Design review of the part built by this model. Coordinates are the model's own, in mm. A direction names the side the tool comes from. Round coordinates to 2 decimals unless told otherwise and drop trailing zeros. Order: outer loops, then holes, each group sorted by start corner. A loop starts at its lowest first (then second) coordinate and runs counter-clockwise, first axis right, second up. Notation, with made-up numbers: M 41,45.5 L 80,45.5 A26 ccw 80,65.5 Z; hole C 85.5,-5 d7. An arc over 180 degrees is marked long. Use a Markdown table: item, result. Add a question column.
(1) Take a section at A-A (z = -232.5). Write out the cut boundary in (x, y), then the cut area to 3 significant figures.
(2) Machinability: for faces 4 (the face through (0.986, 5.768, -155.615)), 5 (the face through (2, -11, -148)), which of the approach directions +Z, -Z, +X, -X, +Y, -Y give a long, thin tool a straight path to every point of the face, cutting with its end or side? Answer none if there is none.
(3) The part is to be moulded in two halves that separate along Z. For faces 1 (the face through (0.99, 24, -317.23)), 2 (the face through (0, -11, -148)), 3 (the face through (0.99, 27.33, -155.99)), say which applies: released by +Z, released by -Z, zero draft, split by the parting line, or undercut.
(4) To check wall thickness, follow probe 1 along Y at (x, z) = (1.9, -175.5); probe 2 along Z at (x, y) = (1.1, 35); probe 3 along Z at (x, y) = (1.9, -18.5). State the ranges of each line that lie inside material, in increasing order. Write a range as from..to.
(5) For pin 1 (0.6 mm diameter, centred on x = 1, y = -8, fed in from +Z); pin 2 (0.6 mm diameter, centred on x = 1, y = -49.5, fed in from -Z); pin 3 (0.6 mm diameter, centred on x = 1, z = -118.5, fed in from -Y), all flat-tipped, find the tip position at first contact; note any pin that passes through.
(6) Take a section at B-B (z = -116). Write out the cut boundary in (x, y), then the cut area to 3 significant figures.
(7) Take a section at C-C (x = 1.7). Count the separate pieces of the cut face and the enclosed holes in it, then the cut area to 3 significant figures.
```python
from build123d import *

# Parameters (mm, degrees)
SKETCH_1_W          = 40
SKETCH_1_H          = 2
SKETCH_1_W_2        = 50
SKETCH_1_R          = 15
SKETCH_1_W_3        = 30
SKETCH_1_W_4        = 2
SKETCH_1_H_2        = 40
EXTRUDE_3_DEPTH     = 2
SKETCH_2_W          = 190.078492772
SKETCH_2_H          = 26.673691145
EXTRUDE_4_DEPTH     = 2
CUT_EXTRUDE_1_DEPTH = 2
CUT_EXTRUDE_2_DEPTH = 2


with BuildPart() as part:
    # 草图1 → 凸台-拉伸3 (new body)
    # profile 1 of 4: a face of its own
    with BuildSketch(Plane(origin=(0, 0, 0), x_dir=(0, 0, -1), z_dir=(1, 0, 0))):
        Polygon((139, 51), (0, 51), (0, 20), (2, 20), (2, -20), (0, -20), (0, -51), (100, -51), (100, -49), (140, -49), (140, -51), (350, -51), (350, -20), (350, 20), (350, 51), (337.5, 51), (331.5, 51), (145, 51), align=None)
        with Locations((59.999999544, -18.999999639)):
            Rectangle(SKETCH_1_W, SKETCH_1_H, mode=Mode.SUBTRACT)
        with BuildLine():
            Line((145, -43), (145, -32))
            ThreePointArc((145, -32), (146.757359313, -27.757359313), (151, -26))
            Line((151, -26), (235, -26))
            Line((235, -26), (305, -26))
            Line((305, -26), (325.5, -26))
            ThreePointArc((325.5, -26), (329.742640687, -27.757359313), (331.5, -32))
            Line((331.5, -32), (331.5, -35))
            Line((331.5, -35), (331.5, -43))
            ThreePointArc((331.5, -43), (329.742640687, -47.242640687), (325.5, -49))
            Line((325.5, -49), (151, -49))
            ThreePointArc((151, -49), (146.757359313, -47.242640687), (145, -43))
        make_face(mode=Mode.SUBTRACT)
        with Locations((174.999999544, -18.999999639)):
            Rectangle(SKETCH_1_W_2, SKETCH_1_H, mode=Mode.SUBTRACT)
        with Locations((294.999999544, -18.999999639)):
            Rectangle(SKETCH_1_W_2, SKETCH_1_H, mode=Mode.SUBTRACT)
        with BuildLine():
            Line((35.191745107, 4.260800891), (35.191745107, 29.047933032))
            ThreePointArc((35.191745107, 29.047933032), (35.944654017, 30.348646261), (37.447551645, 30.343601384))
            Line((37.447551645, 30.343601384), (58.776761499, 17.901562302))
            ThreePointArc((58.776761499, 17.901562302), (59.520952796, 16.603345479), (58.772354511, 15.307664881))
            Line((58.772354511, 15.307664881), (37.443144656, 2.962571821))
            ThreePointArc((37.443144656, 2.962571821), (35.942445208, 2.961358833), (35.191745107, 4.260800891))
        make_face(mode=Mode.SUBTRACT)
        with BuildLine():
            Line((89.643364252, -3.340511469), (45.740125962, -3.340511469))
            ThreePointArc((45.740125962, -3.340511469), (44.292109641, -2.231981438), (44.984319423, -0.544843118))
            Line((44.984319423, -0.544843118), (66.935938568, 12.26026805))
            ThreePointArc((66.935938568, 12.26026805), (67.691745107, 12.464599699), (68.447551645, 12.26026805))
            Line((68.447551645, 12.26026805), (90.39917079, -0.544843118))
            ThreePointArc((90.39917079, -0.544843118), (91.091380572, -2.231981438), (89.643364252, -3.340511469))
        make_face(mode=Mode.SUBTRACT)
        with BuildLine():
            ThreePointArc((97.935938568, 30.343601384), (99.438836196, 30.348646261), (100.191745107, 29.047933032))
            Line((100.191745107, 29.047933032), (100.191745107, 4.27104403))
            ThreePointArc((100.191745107, 4.27104403), (99.438836196, 2.970330801), (97.935938568, 2.975375678))
            Line((97.935938568, 2.975375678), (76.698605138, 15.36382018))
            ThreePointArc((76.698605138, 15.36382018), (75.954411676, 16.659488531), (76.698605138, 17.955156882))
            Line((76.698605138, 17.955156882), (97.935938568, 30.343601384))
        make_face(mode=Mode.SUBTRACT)
        with BuildLine():
            Line((134.999999544, 4.260800891), (134.999999544, 29.047933032))
            ThreePointArc((134.999999544, 29.047933032), (135.752908454, 30.348646261), (137.255806082, 30.343601384))
            Line((137.255806082, 30.343601384), (158.585015936, 17.901562302))
            ThreePointArc((158.585015936, 17.901562302), (159.329207233, 16.603345479), (158.580608948, 15.307664881))
            Line((158.580608948, 15.307664881), (137.251399093, 2.962571821))
            ThreePointArc((137.251399093, 2.962571821), (135.750699645, 2.961358833), (134.999999544, 4.260800891))
        make_face(mode=Mode.SUBTRACT)
        with BuildLine():
            ThreePointArc((44.984319423, 33.86382018), (44.292109641, 35.5509585), (45.740125962, 36.659488531))
            Line((45.740125962, 36.659488531), (90.076890905, 36.659488531))
            ThreePointArc((90.076890905, 36.659488531), (91.525570236, 35.548497783), (90.828290455, 33.861259462))
            Line((90.828290455, 33.861259462), (68.573204266, 20.980280188))
            ThreePointArc((68.573204266, 20.980280188), (67.819256245, 20.778511422), (67.065998178, 20.982840906))
            Line((67.065998178, 20.982840906), (44.984319423, 33.86382018))
        make_face(mode=Mode.SUBTRACT)
        with BuildLine():
            Line((189.451618689, -3.340511469), (145.548380399, -3.340511469))
            ThreePointArc((145.548380399, -3.340511469), (144.100364078, -2.231981438), (144.79257386, -0.544843118))
            Line((144.79257386, -0.544843118), (166.744193005, 12.26026805))
            ThreePointArc((166.744193005, 12.26026805), (167.499999544, 12.464599699), (168.255806082, 12.26026805))
            Line((168.255806082, 12.26026805), (190.207425227, -0.544843118))
            ThreePointArc((190.207425227, -0.544843118), (190.899635009, -2.231981438), (189.451618689, -3.340511469))
        make_face(mode=Mode.SUBTRACT)
        with BuildLine():
            ThreePointArc((197.744193005, 30.684113214), (199.247090633, 30.689158091), (199.999999544, 29.388444862))
            Line((199.999999544, 29.388444862), (199.999999544, 4.61155586))
            ThreePointArc((199.999999544, 4.61155586), (199.247090633, 3.310842631), (197.744193005, 3.315887508))
            Line((197.744193005, 3.315887508), (176.506859575, 15.70433201))
            ThreePointArc((176.506859575, 15.70433201), (175.762666113, 17.000000361), (176.506859575, 18.295668712))
            Line((176.506859575, 18.295668712), (197.744193005, 30.684113214))
        make_face(mode=Mode.SUBTRACT)
        with Locations((232.499999544, 17.000000361)):
            Circle(SKETCH_1_R, mode=Mode.SUBTRACT)
        with BuildLine():
            Line((319.974166341, -3.394327578), (276.070928051, -3.394327578))
            ThreePointArc((276.070928051, -3.394327578), (274.622911731, -2.285797546), (275.315121513, -0.598659226))
            Line((275.315121513, -0.598659226), (297.266740658, 12.206451942))
            ThreePointArc((297.266740658, 12.206451942), (298.022547196, 12.41078359), (298.778353734, 12.206451942))
            Line((298.778353734, 12.206451942), (320.729972879, -0.598659226))
            ThreePointArc((320.729972879, -0.598659226), (321.422182661, -2.285797546), (319.974166341, -3.394327578))
        make_face(mode=Mode.SUBTRACT)
        with BuildLine():
            Line((265.522547196, 4.206984782), (265.522547196, 28.994116924))
            ThreePointArc((265.522547196, 28.994116924), (266.275456106, 30.294830153), (267.778353734, 30.289785275))
            Line((267.778353734, 30.289785275), (289.107563589, 17.847746193))
            ThreePointArc((289.107563589, 17.847746193), (289.851754885, 16.549529371), (289.1031566, 15.253848773))
            Line((289.1031566, 15.253848773), (267.773946745, 2.908755713))
            ThreePointArc((267.773946745, 2.908755713), (266.273247297, 2.907542724), (265.522547196, 4.206984782))
        make_face(mode=Mode.SUBTRACT)
        with BuildLine():
            ThreePointArc((327.730104048, 30.281463391), (329.239984934, 30.298885724), (329.999999544, 28.994116924))
            Line((329.999999544, 28.994116924), (329.999999544, 4.522047385))
            ThreePointArc((329.999999544, 4.522047385), (329.247090633, 3.221334156), (327.744193005, 3.226379034))
            Line((327.744193005, 3.226379034), (307.029407227, 15.310004071))
            ThreePointArc((307.029407227, 15.310004071), (306.285236078, 16.597490851), (307.01531827, 17.893018889))
            Line((307.01531827, 17.893018889), (327.730104048, 30.281463391))
        make_face(mode=Mode.SUBTRACT)
        with BuildLine():
            ThreePointArc((144.79257386, 33.86382018), (144.100364078, 35.5509585), (145.548380399, 36.659488531))
            Line((145.548380399, 36.659488531), (189.885145343, 36.659488531))
            ThreePointArc((189.885145343, 36.659488531), (191.333824673, 35.548497783), (190.636544892, 33.861259462))
            Line((190.636544892, 33.861259462), (168.381458703, 20.980280188))
            ThreePointArc((168.381458703, 20.980280188), (167.627510682, 20.778511422), (166.874252615, 20.982840906))
            Line((166.874252615, 20.982840906), (144.79257386, 33.86382018))
        make_face(mode=Mode.SUBTRACT)
        with BuildLine():
            ThreePointArc((275.298058871, 34.214436971), (274.625531032, 35.901033349), (276.070928051, 37.000000361))
            Line((276.070928051, 37.000000361), (321.088992302, 37.000000361))
            ThreePointArc((321.088992302, 37.000000361), (322.537671633, 35.889009613), (321.840391852, 34.201771291))
            Line((321.840391852, 34.201771291), (298.904006355, 20.926464079))
            ThreePointArc((298.904006355, 20.926464079), (298.140143214, 20.72474493), (297.379737626, 20.939129758))
            Line((297.379737626, 20.939129758), (275.298058871, 34.214436971))
        make_face(mode=Mode.SUBTRACT)
    # profile 2 of 4: a face of its own
    with BuildSketch(Plane(origin=(0, 0, 0), x_dir=(0, 0, -1), z_dir=(1, 0, 0))):
        with BuildLine():
            Line((0, 20), (0, 51))
            ThreePointArc((0, 51), (-36.062445841, 36.062445841), (-51, 0))
            Line((-51, 0), (0, 0))
            Line((0, 0), (0, 20))
        make_face()
        Polygon((-38.821768829, 18.383902445), (-40, 20), (-9.698170842, 42.091834457), (-8.519939671, 40.475736902), align=None, mode=Mode.SUBTRACT)
    # profile 3 of 4: a face of its own
    with BuildSketch(Plane(origin=(0, 0, 0), x_dir=(0, 0, -1), z_dir=(1, 0, 0))):
        with BuildLine():
            Line((0, 0), (-51, 0))
            ThreePointArc((-51, 0), (-36.062445841, -36.062445841), (0, -51))
            Line((0, -51), (0, -20))
            Line((0, -20), (0, 0))
        make_face()
        Polygon((-40, -20), (-38.821768829, -18.383902445), (-8.519939671, -40.475736902), (-9.698170842, -42.091834457), align=None, mode=Mode.SUBTRACT)
        with Locations((-25, -9)):
            Rectangle(SKETCH_1_W_3, SKETCH_1_H, mode=Mode.SUBTRACT)
    # profile 4 of 4: a face of its own
    with BuildSketch(Plane(origin=(0, 0, 0), x_dir=(0, 0, -1), z_dir=(1, 0, 0))):
        with Locations((351, 0)):
            Rectangle(SKETCH_1_W_4, SKETCH_1_H_2)
    extrude(amount=EXTRUDE_3_DEPTH)

    # 草图2 → 凸台-拉伸4 (add)
    with BuildSketch(Plane(origin=(2, 0, 0), x_dir=(0, 0, -1), z_dir=(1, 0, 0))):
        with Locations((237.791738903, -36.733598544)):
            Rectangle(SKETCH_2_W, SKETCH_2_H)
    extrude(amount=-EXTRUDE_4_DEPTH)

    # 草图3 → 切除-拉伸1 (cut)
    with BuildSketch(Plane.ZY):
        Polygon((-276.474715487, -34.635525304), (-276.486854743, -34.329149941), (-274.488422813, -34.249967741), (-273.909339591, -48.865100933), (-275.910680122, -48.870874702), align=None)
        Polygon((-291.918118303, -49), (-292.352577698, -38.034940321), (-292.366784403, -37.676385824), (-290.368352473, -37.597203626), (-289.916778482, -48.994208323), align=None)
    extrude(amount=-CUT_EXTRUDE_1_DEPTH, mode=Mode.SUBTRACT)

    # 草图4 → 切除-拉伸2 (cut)
    with BuildSketch(Plane(origin=(2, 0, 0), x_dir=(0, 0, -1), z_dir=(1, 0, 0))):
        with BuildLine():
            ThreePointArc((167.635934129, -44.518280263), (171.92449544, -40.687294754), (167.952486385, -36.529007588))
            ThreePointArc((167.952486385, -36.529007588), (163.663925074, -40.359993097), (167.635934129, -44.518280263))
        make_face()
    extrude(amount=-CUT_EXTRUDE_2_DEPTH, mode=Mode.SUBTRACT)


solid = part.part
```
Verdict:
| question | item | result |
|---|---|---|
| 1 | outline | M 0,-51 L 2,-51 L 2,2 L 0,2 Z; M 0,32 L 2,32 L 2,51 L 0,51 Z |
| 1 | area | 144 mm^2 |
| 2 | face 4 | +X, -X |
| 2 | face 5 | +Z, -Z, +X, +Y, -Y |
| 3 | face 1 | undercut |
| 3 | face 2 | zero draft |
| 3 | face 3 | undercut |
| 4 | probe 1 | y = -51..-20, -18..-3.34, 8.03..25.1, 36.66..51 |
| 4 | probe 2 | z = -350..-322.5, -274.66..-191.38, -144.06..-91.57, -44.25..16.03, 19.43..37.09 |
| 4 | probe 3 | z = -352..-320, -270..-200, -150..-80, -40..-2, 0..38.66, 38.91..47.53 |
| 5 | pin 1 | stops at z = 50.42 |
| 5 | pin 2 | stops at z = -350 |
| 5 | pin 3 | stops at y = -49 |
| 6 | outline | M 0,-49 L 2,-49 L 2,51 L 0,51 Z |
| 6 | area | 200 mm^2 |
| 7 | separate pieces | 1 |
| 7 | enclosed holes | 23 |
| 7 | area | 33,500 mm^2 |
